Read the model definition and answer for the solid it produces. Units are mm, in the model's axes. A direction names the side the tool comes from. Give positions to 0.01 mm unless a question says otherwise; leave off trailing zeros. Order: outer loops, then holes, each group sorted by start corner. A loop starts at its lowest first (then second) coordinate and runs counter-clockwise, first axis right, second up. Notation, with made-up numbers: (-33, 83) - (-8, 83) arc R16 cw to (-8, 110) - close; hole circle Ø10 at (74.5, -31). An arc over 180 degrees is marked (long way). Use a Markdown table: item, result. Add a question column.
1. For a pull along Z with two mould halves and no side action, classify faces 3 (the flat face through (36, 0, 900)), 4 (the flat face through (36, 0, -900)), 5 (the flat face through (25, 0, 12)), 6 (the flat face through (-25, 0, 12)) as released by +Z, released by -Z, zero draft, split by the parting line, or undercut.
2. Consider L1, parallel to Z at x = 37, y = 18; L2, parallel to X at y = -21.5, z = 116; L3, parallel to Z at x = 81, y = -7. Determine where each line is inside the solid, lowest interval first.
3. A cutting plane is placed at B-B on y = 15. Determine the outline of the cut face in (x, z), and give its area (3 significant figures).
4. Which of the six approach directions +Z, -Z, +X, -X, +Y, -Y give full straight-line access (tool end or side, diameter ignored) to faces 1 (the flat face through (8, 25, 13)), 2 (the flat face through (50, 0, -850))?
5. A cutting plane is placed at A-A on x = 59.5. Determine the outline of the cut face in (y, z).
6. Flat-ended cylindrical pins translate along their axes: P1, Ø7.5, axis at x = 83, y = -7, coming from the +Z side; P2, Ø1.5, axis at y = -23.5, z = -403.5, coming from the +X side; P3, Ø10, axis at y = -12, z = 892, coming from the +X side. Find the tip coordinate at first contact, or state that the pin passes through.
7. A cutting plane is placed at C-C on z = 103.5. Determine the outline of the cut face in (x, y).
Autodesk Inventor part; units mm, degrees
ref_plane "YZ Plane" through (0, 0, 0) normal (1, 0, 0) x (0, 1, 0)
ref_plane "XZ Plane" through (0, 0, 0) normal (0, 1, 0) x (-1, 0, 0)
ref_plane "XY Plane" through (0, 0, 0) normal (0, 0, 1) x (1, 0, 0)
sketch "草图1" plane through (0, 0, 0) normal (1, 0, 0) x (0, 1, 0)
  line L0 (-25, 900) -> (25, 900)
  line L1 (25, 900) -> (25, -900)
  line L2 (25, -900) -> (-25, -900)
  line L3 (-25, -900) -> (-25, 900)
  line L4 (-25, 900) -> (25, -900) construction
  line L5 (25, 900) -> (-25, -900) construction
  point P0 (0, 0)
  dimension "d0" = 50
  dimension "d1" = 1800
extrude "拉伸1" add sketch "草图1" against normal mid plane 50
sketch "草图2" plane through (25, 0, 0) normal (1, 0, 0) x (0, 0, -1)
  line L0 (-900, -25) -> (-900, 25)
  line L1 (-900, 25) -> (-850, 25)
  line L2 (-850, 25) -> (-850, -25)
  line L3 (-850, -25) -> (-900, -25)
  line L4 (-900, -25) -> (-900, 25)
  line L5 (-900, 25) -> (900, 25) construction
  line L6 (0, 25) -> (0, -25) construction
  line L7 (900, -25) -> (-900, -25) construction
  line L8 (900, -25) -> (900, 25)
  line L9 (900, 25) -> (850, 25)
  line L10 (850, 25) -> (850, -25)
  line L11 (850, -25) -> (900, -25)
  line L12 (900, -25) -> (900, 25)
  line L13 (900, 25) -> (-900, 25) construction
  line L14 (-900, -25) -> (900, -25) construction
  point P0 (0, 0)
  dimension "d4" = 50
  dimension "d5" = 50
extrude "拉伸2" add sketch "草图2" along normal blind 50
sketch "草图3" plane through (75, 0, 0) normal (1, 0, 0) x (0, 0, -1)
  line L0 (850, 25) -> (850, -25)
  line L1 (850, 25) -> (870, 25)
  line L2 (900, 25) -> (880, 25)
  line L3 (870, 25) -> (880, 25)
  line L4 (880, 25) -> (880, -25)
  line L5 (880, -25) -> (870, -25)
  line L6 (870, -25) -> (870, 25)
  line L7 (0, 25) -> (0, -25) construction
  line L8 (-850, 25) -> (-850, -25)
  line L9 (-850, 25) -> (-870, 25)
  line L10 (-900, 25) -> (-880, 25)
  line L11 (-870, 25) -> (-880, 25)
  line L12 (-880, 25) -> (-880, -25)
  line L13 (-880, -25) -> (-870, -25)
  line L14 (-870, -25) -> (-870, 25)
  line L15 (880, -25) -> (870, -25)
  line L16 (850, -25) -> (900, -25)
  line L17 (-880, -25) -> (-870, -25)
  line L18 (900, -25) -> (-900, -25)
  point P0 (0, 0)
  point P1 (-900, 25)
  point P2 (-850, 25)
  dimension "d10" = 10
  dimension "d11" = 20
extrude "拉伸3" add sketch "草图3" along normal blind 15 contours L3 L4 L5 L6 | L13 L12 L11 L14
sketch "草图4" plane through (-25, -25, -900) normal (0, -1, 0) x (1, 0, 0)
  line L0 (0, 0) -> (20, 0)
  line L1 (100, 0) -> (0, 0)
  line L2 (20, 0) -> (30, 0)
  line L3 (20, 0) -> (25, 0)
  line L4 (25, 0) -> (25, 1800)
  line L5 (25, 1800) -> (20, 1800)
  line L6 (20, 1800) -> (20, 0)
  line L7 (0, 1800) -> (100, 1800)
  point P0 (25, 900)
  dimension "d12" = 20
  dimension "d13" = 10
  dimension "d14" = 5
  dimension "d16" = 1800
extrude "拉伸4" cut sketch "草图4" against normal blind 5
fillet "圆角1" radius 20 2 edges at (-25, 0, 900) (-25, 0, -900)
properties part number "水平滑台"
Output values:
| question | item | result |
|---|---|---|
| 1 | face 3 | released by +Z |
| 1 | face 4 | released by -Z |
| 1 | face 5 | undercut |
| 1 | face 6 | zero draft |
| 2 | L1 | -900 to -850, 850 to 900 |
| 2 | L2 | -25 to -5, 0 to 25 |
| 2 | L3 | -880 to -870, 870 to 880 |
| 3 | outline | (-25, -880) arc R20 ccw to (-5, -900) - (75, -900) - (75, -880) - (90, -880) - (90, -870) - (75, -870) - (75, -850) - (25, -850) - (25, 850) - (75, 850) - (75, 870) - (90, 870) - (90, 880) - (75, 880) - (75, 900) - (-5, 900) arc R20 ccw to (-25, 880) - close |
| 3 | area | 95,100 mm² |
| 4 | face 1 | +Z, -Z, +X, -X, +Y |
| 4 | face 2 | +X, +Y, -Y |
| 5 | outline | (-25, -900) - (25, -900) - (25, -850) - (-25, -850) - close; (-25, 850) - (25, 850) - (25, 900) - (-25, 900) - close |
| 6 | P1 | z = 880 |
| 6 | P2 | x = 25 |
| 6 | P3 | x = 75 |
| 7 | outline | (-25, -25) - (-5, -25) - (-5, -20) - (0, -20) - (0, -25) - (25, -25) - (25, 25) - (-25, 25) - close |
